Can you work these out from the model? Positions are in its coordinate system, mm. A direction names the side the tool comes from. Give positions to 0.01 mm unless a question says otherwise; leave off trailing zeros. Loops run counter-clockwise (first coordinate to the right, second up) from the corner with the lowest first, then second, coordinate; pieces in that order, holes last. Notation, with made-up numbers: (69, -37.75) -> (107, -37.75) arc R20 cw to (107, -24.75) -> close; hole circle Ø8 at (56, 15). An arc over 180 degrees is marked (long way). Return JSON: item names as keys, results as strings. Group by question number.
Q1. Suppose I cut it at C-C, the plane x = -3.5. Please give me the cut outline in (y, z).
Q2. Which directions (+Z, -Z, +X, -X, +Y, -Y) give clear straight access to the entire face, cutting with the end or side of a thin tool? Please do faces 1 (the flat face through (-11.796, 5, 24)), 2 (the flat face through (1.204, 5, 25)), 3 (the flat face through (-5, 0, 16)).
Q3. Will these pins go through, and if not, where does the flat tip stop? pin 1 (3 mm diameter, centred on y = 7, z = -29, fed in from -X); pin 2 (2 mm diameter, centred on y = 2.5, z = 35.5, fed in from +X); pin 3 (5 mm diameter, centred on x = -3, y = 3.5, fed in from -Z); pin 4 (6 mm diameter, centred on x = -12.5, y = 7, fed in from +Z).
Q4. Suppose I cut it at A-A, the plane y = 8. Please give me the cut outline in (x, z).
Q5. Suppose I cut it at B-B, the plane z = 13. Please give me the cut outline in (x, y), and give its area (3 significant figures).
Q6. I need wall thicknesses on line 1 along X through (y, z) = (1.5, 74); line 2 along Z through (x, y) = (-0.75, 5.25); line 3 along Z through (x, y) = (-5.5, 4). Which ranges of each line are inside material? Lowest first, please. Write a range as [from, to].
```python
from build123d import *

# Parameters (mm, degrees)
ESTRUSIONE_ESTRUSIONE1_DEPTH = 10
TAGLIO_ESTRUSIONE1_DEPTH     = 85.287841486


with BuildPart() as part:
    # Schizzo1 → Estrusione-Estrusione1 (new body)
    with BuildSketch(Plane(origin=(0, 0, 0), x_dir=(1, 0, 0), z_dir=(0, 1, 0))):
        with BuildLine():
            ThreePointArc((1.203512806, 33.499091111), (-5.296487194, 30.981587168), (-11.796487194, 33.499091111))
            Line((-11.796487194, 33.499091111), (-11.796487194, -82.347087033))
            Line((-11.796487194, -82.347087033), (1.203512806, -82.347087033))
            Line((1.203512806, -82.347087033), (1.203512806, 33.499091111))
        make_face()
        with BuildLine():
            ThreePointArc((1.203512806, 37.652912967), (-5.296487194, 33.481587168), (-11.796487194, 37.652912967))
            Line((-11.796487194, 37.652912967), (-11.796487194, 33.499091111))
            ThreePointArc((-11.796487194, 33.499091111), (-5.296487194, 30.981587168), (1.203512806, 33.499091111))
            Line((1.203512806, 33.499091111), (1.203512806, 37.652912967))
        make_face()
        with BuildLine():
            Line((-11.796487194, 33.499091111), (-11.796487194, 37.652912967))
            ThreePointArc((-11.796487194, 37.652912967), (-6.820872316, 47.617197378), (1.853512806, 40.631587168))
            ThreePointArc((1.853512806, 40.631587168), (1.689123016, 39.107202046), (1.203512806, 37.652912967))
            Line((1.203512806, 37.652912967), (1.203512806, 33.499091111))
            ThreePointArc((1.203512806, 33.499091111), (3.530955811, 36.733029743), (4.353512806, 40.631587168))
            ThreePointArc((4.353512806, 40.631587168), (-9.195044619, 49.459030173), (-11.796487194, 33.499091111))
        make_face()
    extrude(amount=ESTRUSIONE_ESTRUSIONE1_DEPTH)

    # Schizzo2 → Taglio-Estrusione1 (cut, through all)
    with BuildSketch(Plane(origin=(0, 10, 0), x_dir=(1, 0, 0), z_dir=(0, 1, 0))):
        Polygon((-16.367555006, 53.62907886), (5.774580618, 53.62907886), (-1.296487194, 46.558011048), (-9.296487194, 46.558011048), align=None)
    extrude(amount=-TAGLIO_ESTRUSIONE1_DEPTH, mode=Mode.SUBTRACT)


solid = part.part
```
Ans:
{
 "1": {"outline": "(0, -33.71) -> (10, -33.71) -> (10, 82.35) -> (0, 82.35) -> close"},
 "2": {"face 1": "+Z, -X, +Y, -Y", "face 2": "+Z, +X, +Y, -Y", "face 3": "+Z, -Z, +X, -X, -Y"},
 "3": {"pin 1": "stops at x = -11.8", "pin 2": "stops at x = 1.2", "pin 3": "stops at z = -47.35", "pin 4": "stops at z = 82.35"},
 "4": {"outline": "(-11.8, -33.5) arc R9.65 ccw to (-11.09, -48.35) -> (-9.3, -46.56) arc R7.15 cw (long way) to (-1.3, -46.56) -> (0.5, -48.35) arc R9.65 ccw to (1.2, -33.5) -> (1.2, 82.35) -> (-11.8, 82.35) -> close"},
 "5": {"outline": "(-11.8, 0) -> (1.2, 0) -> (1.2, 10) -> (-11.8, 10) -> close", "area": "130 mm^2"},
 "6": {"line 1": "x = [-11.8, 1.2]", "line 2": "z = [-47.1, -46.15], [-35.11, 82.35]", "line 3": "z = [-33.48, 82.35]"}
}
